Input: part model. Units: mm. Frame: model coordinates. A direction names the side the tool comes from. Round coordinates to 2 decimals unless told otherwise and drop trailing zeros. Loops run counter-clockwise (first coordinate to the right, second up) from the corner with the lowest first, then second, coordinate; pieces in that order, holes last.
(1) Cut plane B-B, the plane x = 38.5. Output: boundary loops of the cut face in (y, z), and give its area (3 significant figures).
(2) Cut plane A-A, the plane z = -66. Output: boundary loops of the cut face in (x, y).
(3) Draft query along Y for faces 3 (the face through (-1, -25, -19.05)), 4 (the face through (-4.01, -18.06, -55.35)), 5 (the face through (-2.799, -21.317, -49.733)), 6 (the face through (-8.767, -16.856, -125.146)). Return one class per face: released by +Y, released by -Y, zero draft, split by the parting line, or undercut.
(4) Cut plane C-C, the plane y = 31.5. Output: boundary loops of the cut face in (x, z), and give its area (3 significant figures).
(5) First-contact query: pin 1 Ø10 at (y, z) = (11, -51) entering from -X; pin 2 Ø2 at (x, y) = (0, 21.21) entering from +Z; pin 3 Ø2 at (y, z) = (-23.5, -31.5) entering from +X; pin 4 Ø11 at (x, y) = (30.08, -41.41) entering from -Z. Flat tips, straight axial feed; report the tip coordinate or a pass-through.
(6) Line query: line 1 (Y direction, x = 15, z = -4); line 2 (X direction, y = -15, z = -5); line 3 (X direction, y = 19, z = -13.5). Output: solid intervals per line, ascending.
(7) Cut plane D-D, the plane z = -93. Output: boundary loops of the cut face in (x, y).
(8) Access query for faces 1 (the face through (-31.282, 37.364, -9.392)), 2 (the face through (-4.1, -18.2, -112.268)). Directions: +Z, -Z, +X, -X, +Y, -Y. A direction counts if a zero-diameter tool reaches every point of the face in a straight line with its end or side. Return the directions, or none.
from build123d import *

# Parameters (mm, degrees)
SKETCH1_R                 = 19.5
SKETCH1_R_2               = 18.5
EXTRUDE1_DEPTH            = 137.668
SKETCH4_R                 = 57.15
SKETCH4_R_2               = 19.5
EXTRUDE2_DEPTH            = 19.05
CUT_EXTRUDE1_REACH        = 161.639
SKETCH5_R                 = 4.2164
CIRPATTERN1_COUNT         = 10
F_4_40_TAPPED_HOLE2_D     = 2.2606
F_4_40_TAPPED_HOLE2_DEPTH = 7.62
F_4_40_TAPPED_HOLE2_TIP   = 0.679152758
SKETCH10_R                = 19
EXTRUDE3_DEPTH            = 25.4
EXTRUDE4_START            = 63
SKETCH12_R                = 21.5
SKETCH12_R_2              = 19
EXTRUDE4_DEPTH            = 63
FILLET1_R                 = 2.54
FILLET2_R                 = 2.54


with BuildPart() as part:
    # Sketch1 → Extrude1 (new body)
    with BuildSketch(Plane.XY):
        Circle(SKETCH1_R)
        Circle(SKETCH1_R_2, mode=Mode.SUBTRACT)
    extrude(amount=-EXTRUDE1_DEPTH)

    # Sketch4 → Extrude2 (add)
    with BuildSketch(Plane.XY):
        Circle(SKETCH4_R)
        Circle(SKETCH4_R_2, mode=Mode.SUBTRACT)
    extrude(amount=-EXTRUDE2_DEPTH)

    # Sketch5 → Cut-Extrude1 (cut, up to next)
    with BuildSketch(Plane.XY, mode=Mode.PRIVATE) as cut_extrude1_sk1:
        with Locations((0, 51.181)):
            Circle(SKETCH5_R)
    cut_extrude1_tool1 = extrude(cut_extrude1_sk1.sketch, amount=-CUT_EXTRUDE1_REACH, mode=Mode.PRIVATE) & part.part
    cut_extrude1 = cut_extrude1_tool1.solids().sort_by_distance((0, 51.181, 0))[0]
    add(cut_extrude1, mode=Mode.SUBTRACT)

    # CirPattern1: Cut-Extrude1 ×10 about axis
    cirpattern1_axis = Axis((0, 0, 0), (0, 0, 1))
    for i in range(1, CIRPATTERN1_COUNT):
        add(cut_extrude1.rotate(cirpattern1_axis, i * 360 / CIRPATTERN1_COUNT), mode=Mode.SUBTRACT)

    # #4-40 Tapped Hole2
    with Locations(Plane.XY):
        with Locations((15, -15), (-15, -15), (-15, 15), (15, 15), (0, 21.213203436), (-21.213203436, 0), (21.213203436, 0), (0, -21.213203436)):
            Hole(F_4_40_TAPPED_HOLE2_D / 2, depth=F_4_40_TAPPED_HOLE2_DEPTH)
            with Locations((0, 0, -(F_4_40_TAPPED_HOLE2_DEPTH + F_4_40_TAPPED_HOLE2_TIP / 2))):  # 118° drill point
                Cone(0, F_4_40_TAPPED_HOLE2_D / 2, F_4_40_TAPPED_HOLE2_TIP, mode=Mode.SUBTRACT)

    # Sketch10 → Extrude3 (cut)
    with BuildSketch(Plane(origin=(0, 0, -137.668), x_dir=(-1, 0, 0), z_dir=(0, 0, -1))):
        Circle(SKETCH10_R)
    extrude(amount=-EXTRUDE3_DEPTH, mode=Mode.SUBTRACT)

    # Sketch12 → Extrude4 (add)
    with BuildSketch(Plane(origin=(0, 0, -19.05), x_dir=(-1, 0, 0), z_dir=(0, 0, -1)).offset(EXTRUDE4_START)):
        with Locations(Location((0, 0, 0), (0, 0, 180))):
            Circle(SKETCH12_R)
        Circle(SKETCH12_R_2, mode=Mode.SUBTRACT)
    extrude(amount=-EXTRUDE4_DEPTH)

    # Fillet1
    # the kernel refuses this fillet: 2.54 mm, written as the material it takes off along each edge
    with BuildSketch(Plane(origin=(0, 0, -82.05), x_dir=(1, 0, 0), z_dir=(0, 1, 0))) as fillet1_piece_1:
        with BuildLine():
            CenterArc((18.96, -2.481934729), FILLET1_R, 0, 77.725329785)
            Line((21.5, -2.481934729), (21.5508, -2.481934729))
            Line((21.5508, -2.481934729), (21.5508, 0))
            Line((21.5508, 0), (21.5, 0.0508))
            ThreePointArc((21.5, 0.0508), (20.5, 0.0508), (19.5108, 0.049638695))
            Line((19.5108, 0.049638695), (19.5, 0))
        make_face()
    revolve(axis=Axis((0, 0, -82.05), (0, 0, -1)), mode=Mode.SUBTRACT)

    # Fillet2
    fillet2_edges = [part.edges().sort_by_distance(p)[0] for p in [
        (-19.5, 0, -82.05),
    ]]
    fillet(fillet2_edges, radius=FILLET2_R)


solid = part.part
Reported:
1. outline: (-42.24, -19.05) - (42.24, -19.05) - (42.24, 0) - (-42.24, 0) - close
1. area: 1,610 mm2
2. outline: circle Ø43 at (0, 0); hole circle Ø37 at (0, 0)
3. face 3: zero draft
3. face 4: undercut
3. face 5: split by the parting line
3. face 6: undercut
4. outline: (-47.69, -19.05) - (47.69, -19.05) - (47.69, 0) - (-47.69, 0) - close
4. area: 1,820 mm2
5. pin 1: stops at x = -20.65
5. pin 2: stops at z = -7.7
5. pin 3: passes through
5. pin 4: stops at z = -19.05
6. line 1: y = -55.15 to -16.13, -13.87 to -10.83, 10.83 to 13.87, 16.13 to 55.15
6. line 2: x = -55.15 to -52.81, -44.54 to -16.13, -13.87 to -10.83, 10.83 to 13.87, 16.13 to 44.54, 52.81 to 55.15
6. line 3: x = -53.9 to -51.44, -45.91 to 45.91, 51.44 to 53.9
7. outline: circle Ø39 at (0, 0); hole circle Ø37 at (0, 0)
8. face 1: +Z, -Z
8. face 2: -Z
